Autodesk Inventor part; units mm, degrees
ref_plane "YZ Plane" through (0, 0, 0) normal (1, 0, 0) x (0, 1, 0)
ref_plane "XZ Plane" through (0, 0, 0) normal (0, 1, 0) x (-1, 0, 0)
ref_plane "XY Plane" through (0, 0, 0) normal (0, 0, 1) x (1, 0, 0)
sketch "Sketch1" plane through (0, 0, 0) normal (0, 0, 1) x (1, 0, 0)
  line L0 (0, 0) -> (0, 68.7718)
  line L1 (0, 0) -> (-35.2548, 0) construction
  line L2 (-25.4, 0) -> (-25.4, 73.68)
  line L3 (-25.4, 73.68) -> (-12.7, 110.52)
  line L4 (-12.7, 110.52) -> (-12.7, 184.2)
  line L5 (-11.05, 184.2) -> (-11.05, 110.2436)
  line L6 (-11.05, 110.2436) -> (-23.75, 73.4036)
  line L7 (-23.75, 73.4036) -> (-23.75, 0)
  line L8 (-25.4, 0) -> (-23.75, 0)
  line L9 (-12.7, 184.2) -> (-11.05, 184.2)
  dimension "d0" = 1.65
  dimension "d1" = 25.4
  dimension "d2" = 73.68
  dimension "d3" = 73.68
  dimension "d4" = 184.2
  dimension "d5" = 50.8
revolve "Revolution1" add sketch "Sketch1" angle 360 about axis through (0, 0, 0) along (0, 1, 0)
equation "\"d2\" = 0.4 * d4"
equation "\"d3\" = d2"
properties part number "ASME BPE CON RED-50.8-25.4"
Geometry check sheet. Reference: the model listing, model coordinates, mm. A direction names the side the tool comes from. Coordinates: 2 decimals unless noted, no trailing zeros. Order: outer loops, then holes, each group sorted by start corner. A loop starts at its lowest first (then second) coordinate and runs counter-clockwise, first axis right, second up. Notation, with made-up numbers: (43.5, 55.5) - (61.5, 55.5) arc R31 cw to (61.5, 89.5) - close; hole circle Ø6 at (53.5, -14). An arc over 180 degrees is marked (long way). Answer as a JSON object with one key per item and string values. Group by question number.
Item 1: Depth check by flat-ended pin: pin 1 Ø12 at (y, z) = (23.5, -4.5) entering from +X; pin 2 Ø2 at (y, z) = (97.5, 3.5) entering from +X; pin 3 Ø1.5 at (x, y) = (16.5, 46) entering from +Z; pin 4 Ø2 at (x, y) = (18, 82) entering from +Z. Enter the tip coordinate at first touch or a pass-through.
Item 2: Scan lines: probe 1 along Z at (x, y) = (0, 45); probe 2 along Z at (x, y) = (0, 138); probe 3 along X at (y, z) = (72, 5). Record each from-to range of solid material in increasing order.
Item 3: Sectioned sample at C-C, the plane y = 172.5. Record the cut outline in (x, z).
Item 4: Sectioned sample at A-A, the plane x = 0. Record the cut outline in (y, z), and give its area (3 significant figures).
Item 5: Tool access check on faces 4 (the face through (1, 184.2, -11.2)), 5 (the face through (5.149, 36.188, 23.185)). Record the directions out of +Z, -Z, +X, -X, +Y, -Y that give a thin tool (end or side, any length) a straight path to the whole face; none if there is none.
Item 6: Sectioned sample at B-B, the plane z = 0. Record the cut outline in (x, y), and give its area (3 significant figures).
Item 7: Draft check along X on faces 1 (the face through (2.75, 147.88, -12.4)), 2 (the face through (2.395, 146.704, 10.787)), 3 (the face through (-17, 0, -17)). Enter one of: +X half, -X half, draft (parallel to the pull), parting line (faces both ways), or undercut.
Item 8: Sectioned sample at D-D, the plane y = 56.5. Record the cut outline in (x, z), and give its area (3 significant figures).
Resolved:
{
 "1": {"pin 1": "x = 25.4", "pin 2": "x = 17.23", "pin 3": "z = 19.93", "pin 4": "z = 14.9"},
 "2": {"probe 1": "-25.4 to -23.75, 23.75 to 25.4", "probe 2": "-12.7 to -11.05, 11.05 to 12.7", "probe 3": "-24.9 to -23.22, 23.22 to 24.9"},
 "3": {"outline": "circle Ø25.4 at (0, 0); hole circle Ø22.1 at (0, 0)"},
 "4": {"outline": "(0, -25.4) - (73.68, -25.4) - (110.52, -12.7) - (184.2, -12.7) - (184.2, -11.05) - (110.24, -11.05) - (73.4, -23.75) - (0, -23.75) - close; (0, 23.75) - (73.4, 23.75) - (110.24, 11.05) - (184.2, 11.05) - (184.2, 12.7) - (110.52, 12.7) - (73.68, 25.4) - (0, 25.4) - close", "area": "615 mm^2"},
 "5": {"face 4": "+Z, -Z, +X, -X, +Y", "face 5": "-Y"},
 "6": {"outline": "(-25.4, 0) - (-23.75, 0) - (-23.75, 73.4) - (-11.05, 110.24) - (-11.05, 184.2) - (-12.7, 184.2) - (-12.7, 110.52) - (-25.4, 73.68) - close; (11.05, 110.24) - (23.75, 73.4) - (23.75, 0) - (25.4, 0) - (25.4, 73.68) - (12.7, 110.52) - (12.7, 184.2) - (11.05, 184.2) - close", "area": "615 mm^2"},
 "7": {"face 1": "parting line", "face 2": "undercut", "face 3": "draft"},
 "8": {"outline": "circle Ø50.8 at (0, 0); hole circle Ø47.5 at (0, 0)", "area": "255 mm^2"}
}
